Autodesk Inventor part; units mm, degrees
ref_plane "YZ Plane" through (0, 0, 0) normal (1, 0, 0) x (0, 1, 0)
ref_plane "XZ Plane" through (0, 0, 0) normal (0, 1, 0) x (-1, 0, 0)
ref_plane "XY Plane" through (0, 0, 0) normal (0, 0, 1) x (1, 0, 0)
sketch "Sketch1" plane through (0, 0, 0) normal (1, 0, 0) x (0, 1, 0)
  line L0 (-12.7, 12.7) -> (12.7, 12.7)
  line L1 (12.7, 12.7) -> (12.7, -12.7)
  line L2 (12.7, -12.7) -> (-12.7, -12.7)
  line L3 (-12.7, -12.7) -> (-12.7, 12.7)
  line L4 (-12.7, 12.7) -> (12.7, -12.7) construction
  line L5 (12.7, 12.7) -> (-12.7, -12.7) construction
  point P0 (0, 0)
  dimension "d0" = 25.4
  dimension "d1" = 25.4
extrude "Extrusion1" add sketch "Sketch1" along normal blind 3
sketch "Sketch2" plane through (3, 0, 0) normal (1, 0, 0) x (0, 0, -1)
  line L0 (12.7, -12.7) -> (12.7, 12.7)
  line L1 (12.7, 12.7) -> (-12.7, 12.7)
  line L2 (-12.7, 12.7) -> (-12.7, -12.7)
  line L3 (-12.7, -12.7) -> (12.7, -12.7)
  line L4 (0, 12.7) -> (0, -12.7)
  circle A0 centre (-6.35, 0) radius 4
  line L5 (-11.85, 3.1754) -> (-6.35, 6.3509)
  line L6 (-6.35, 6.3509) -> (-0.85, 3.1754)
  line L7 (-0.85, 3.1754) -> (-0.85, -3.1754)
  line L8 (-0.85, -3.1754) -> (-6.35, -6.3509)
  line L9 (-6.35, -6.3509) -> (-11.85, -3.1754)
  line L10 (-11.85, -3.1754) -> (-11.85, 3.1754)
  circle A1 centre (6.35, 0) radius 4
  line L11 (11.85, 3.1754) -> (6.35, 6.3509)
  line L12 (6.35, 6.3509) -> (0.85, 3.1754)
  line L13 (0.85, 3.1754) -> (0.85, -3.1754)
  line L14 (0.85, -3.1754) -> (6.35, -6.3509)
  line L15 (6.35, -6.3509) -> (11.85, -3.1754)
  line L16 (11.85, -3.1754) -> (11.85, 3.1754)
  point P0 (0, 0)
  point P1 (0, 0)
  point P2 (-0.85, 0)
  point P3 (0.85, 0)
  dimension "d4" = 8
  dimension "d5" = 6.35
  dimension "d6" = 11
extrude "Extrusion2" cut sketch "Sketch2" against normal blind 3 contours A0 | A1
chamfer "Chamfer1" distance 5 angle 45 4 edges at (1.5, -12.7, -12.7) (1.5, -12.7, 12.7) (1.5, 12.7, 12.7) (1.5, 12.7, -12.7)
properties part number "ACOPLE_TORNILLO_DOBLE" material "Steel, Mild, Welded"
Work out the finished part from the listing and answer in its coordinate system (mm). Coordinates: 2 decimals unless noted, no trailing zeros. Order: outer loops, then holes, each group sorted by start corner. A loop starts at its lowest first (then second) coordinate and runs counter-clockwise, first axis right, second up. Notation, with made-up numbers: (21.25, 65.5) - (46.25, 65.5) arc R15 cw to (46.25, 93.5) - close; hole circle Ø10 at (-16, 57.5). An arc over 180 degrees is marked (long way). Put each result on its own line as item: value. Start each with the question number.
1) Find section D-D (y = -9). Give the vertices of the cut face in (x, z).
2) Find section B-B (x = 1.8). Give the vertices of the cut face in (y, z).
3) For a pull along Y with two mould halves and no side action, classify faces 1 (the flat face through (1.5, -10.2, 10.2)), 2 (the cylindrical face through (1.521, -3.905, 7.217)), 3 (the cylindrical face through (1.521, -1.532, -10.045)), 4 (the flat face through (1.5, 10.2, 10.2)) as released by +Y, released by -Y, zero draft, split by the parting line, or undercut.
4) Find section C-C (y = -1). Give the vertices of the cut face in (x, z), plus the area to 3 significant figures.
5) Find section A-A (z = -6.35). Give the vertices of the cut face in (x, y).
6) Find the intervals of material crossed by line 1 (Y direction, x = 2.05, z = 6.35); line 2 (Y direction, x = 2.5, z = -4.25); line 3 (Z direction, x = 2.5, y = 0.5), in increasing order. Write a range as from..to.
Results list:
1. outline: (0, -11.4) - (3, -11.4) - (3, 11.4) - (0, 11.4) - close
2. outline: (-12.7, -7.7) - (-7.7, -12.7) - (7.7, -12.7) - (12.7, -7.7) - (12.7, 7.7) - (7.7, 12.7) - (-7.7, 12.7) - (-12.7, 7.7) - close; hole circle Ø8 at (0, -6.35); hole circle Ø8 at (0, 6.35)
3. face 1: released by -Y
3. face 2: undercut
3. face 3: undercut
3. face 4: released by +Y
4. outline: (0, -12.7) - (3, -12.7) - (3, -10.22) - (0, -10.22) - close; (0, -2.48) - (3, -2.48) - (3, 2.48) - (0, 2.48) - close; (0, 10.22) - (3, 10.22) - (3, 12.7) - (0, 12.7) - close
4. area: 29.7 mm^2
5. outline: (0, -12.7) - (3, -12.7) - (3, -4) - (0, -4) - close; (0, 4) - (3, 4) - (3, 12.7) - (0, 12.7) - close
6. line 1: y = -12.7..-4, 4..12.7
6. line 2: y = -12.7..-3.4, 3.4..12.7
6. line 3: z = -12.7..-10.32, -2.38..2.38, 10.32..12.7
